Can you work these out from the model? Positions are in its coordinate system, mm. A direction names the side the tool comes from. Coordinates: 2 decimals unless noted, no trailing zeros. Loops run counter-clockwise (first coordinate to the right, second up) from the corner with the lowest first, then second, coordinate; pieces in that order, holes last.
Autodesk Inventor part; units mm, degrees
ref_plane "YZ Plane" through (0, 0, 0) normal (1, 0, 0) x (0, 1, 0)
ref_plane "XZ Plane" through (0, 0, 0) normal (0, 1, 0) x (-1, 0, 0)
ref_plane "XY Plane" through (0, 0, 0) normal (0, 0, 1) x (1, 0, 0)
sketch "Skizze1" plane through (0, 0, 0) normal (0, 0, 1) x (1, 0, 0)
  line L0 (48.8, -48.8) -> (-48.8, -48.8)
  line L1 (-48.8, -48.8) -> (-48.8, 48.8)
  line L2 (-48.8, 48.8) -> (48.8, 48.8)
  line L3 (48.8, 48.8) -> (48.8, -48.8)
  line L4 (48.8, -48.8) -> (-48.8, 48.8) construction
  line L5 (-48.8, -48.8) -> (48.8, 48.8) construction
  line L6 (-50, 50) -> (50, 50) construction
  line L7 (50, 50) -> (50, -50) construction
  line L8 (50, -50) -> (-50, -50) construction
  line L9 (-50, -50) -> (-50, 50) construction
  line L10 (-50, 50) -> (50, -50) construction
  line L11 (50, 50) -> (-50, -50) construction
  line L12 (47.75, -47.75) -> (-47.75, -47.75)
  line L13 (-47.75, -47.75) -> (-47.75, 47.75)
  line L14 (-47.75, 47.75) -> (47.75, 47.75)
  line L15 (47.75, 47.75) -> (47.75, -47.75)
  line L16 (47.75, -47.75) -> (-47.75, 47.75) construction
  line L17 (-47.75, -47.75) -> (47.75, 47.75) construction
  circle A0 centre (0, 0) radius 15 construction
  line L18 (-50, 50) -> (-39.5, 50) construction
  line L19 (-39.5, 50) -> (-39.5, 31.5) construction
  line L20 (-39.5, 31.5) -> (-50, 31.5) construction
  line L21 (-50, 31.5) -> (-50, 50) construction
  line L22 (50, 50) -> (39.5, 50) construction
  line L23 (39.5, 50) -> (39.5, 31.5) construction
  line L24 (39.5, 31.5) -> (50, 31.5) construction
  line L25 (50, 31.5) -> (50, 50) construction
  line L26 (-50, -50) -> (-39.5, -50) construction
  line L27 (-39.5, -50) -> (-39.5, -31.5) construction
  line L28 (-39.5, -31.5) -> (-50, -31.5) construction
  line L29 (-50, -31.5) -> (-50, -50) construction
  line L30 (50, -50) -> (39.5, -50) construction
  line L31 (39.5, -50) -> (39.5, -31.5) construction
  line L32 (39.5, -31.5) -> (50, -31.5) construction
  line L33 (50, -31.5) -> (50, -50) construction
  line L34 (-39.5, 47.75) -> (39.5, 47.75)
  line L35 (39.5, 47.75) -> (39.5, 45.75)
  line L36 (39.5, 45.75) -> (-39.5, 45.75)
  line L37 (-39.5, 45.75) -> (-39.5, 47.75)
  line L38 (47.75, 31.5) -> (45.75, 31.5)
  line L39 (45.75, 31.5) -> (45.75, -31.5)
  line L40 (45.75, -31.5) -> (47.75, -31.5)
  line L41 (47.75, -31.5) -> (47.75, 31.5)
  line L42 (39.5, -47.75) -> (-39.5, -47.75)
  line L43 (-39.5, -47.75) -> (-39.5, -45.75)
  line L44 (-39.5, -45.75) -> (39.5, -45.75)
  line L45 (39.5, -45.75) -> (39.5, -47.75)
  line L46 (-47.75, -31.5) -> (-45.75, -31.5)
  line L47 (-45.75, -31.5) -> (-45.75, 31.5)
  line L48 (-45.75, 31.5) -> (-47.75, 31.5)
  line L49 (-47.75, 31.5) -> (-47.75, -31.5)
  line L50 (-39.5, 45.75) -> (-39.5, 31.5)
  line L51 (-45.75, 31.5) -> (-39.5, 31.5)
  line L52 (39.5, 45.75) -> (39.5, 31.5)
  line L53 (39.5, 31.5) -> (45.75, 31.5)
  line L54 (45.75, -31.5) -> (39.5, -31.5)
  line L55 (39.5, -31.5) -> (39.5, -45.75)
  line L56 (-39.5, -45.75) -> (-39.5, -31.5)
  line L57 (-45.75, -31.5) -> (-39.5, -31.5)
  line L58 (-45.75, -29.5) -> (-37.5, -29.5)
  line L59 (-37.5, -29.5) -> (-37.5, -45.75)
  line L60 (45.75, -29.5) -> (37.5, -29.5)
  line L61 (37.5, -29.5) -> (37.5, -45.75)
  line L62 (37.5, 45.75) -> (37.5, 29.5)
  line L63 (37.5, 29.5) -> (45.75, 29.5)
  line L64 (-37.5, 45.75) -> (-37.5, 29.5)
  line L65 (-37.5, 29.5) -> (-45.75, 29.5)
  line L66 (-39.5, 45.75) -> (-37.5, 45.75)
  line L67 (-45.75, 29.5) -> (-45.75, 31.5)
  line L68 (37.5, 45.75) -> (39.5, 45.75)
  line L69 (45.75, 29.5) -> (45.75, 31.5)
  line L70 (45.75, -29.5) -> (45.75, -31.5)
  line L71 (37.5, -45.75) -> (39.5, -45.75)
  line L72 (-39.5, -45.75) -> (-37.5, -45.75)
  line L73 (-45.75, -31.5) -> (-45.75, -29.5)
  point P0 (0, 0)
  point P1 (0, 0)
  point P2 (-10.6066, 10.6066)
  point P3 (10.6066, 10.6066)
  point P4 (10.6066, -10.6066)
  point P5 (-10.6066, -10.6066)
  point P6 (-44, 44)
  point P7 (44, 44)
  point P8 (44, -44)
  point P9 (-44, -44)
  dimension "d0" = 97.6
  dimension "d55" = 30
  dimension "d61" = 100
  dimension "d62" = 95.5
  dimension "d63" = 18.5
  dimension "d64" = 10.5
  dimension "d65" = 2
  dimension "d67" = 6
extrude "Extrusion1" add sketch "Skizze1" against normal blind 2 contours L0 L1 L2 L3 | L12 L45 L55 L54 L40 L15 | L12 L43 L44 L45 | L40 L39 L38 L15 | L12 L13 L46 L57 L56 L43 | L44 L61 L60 L39 L54 L55 | L38 L53 L52 L35 L14 L15 | L56 L57 L47 L58 L59 L44 | L44 L59 L58 L47 L65 L64 L36 L62 L63 L39 L60 L61 | L39 L63 L62 L36 L52 L53 | L13 L48 L47 L46 | L35 L36 L37 L14 | L13 L14 L37 L50 L51 L48 | L51 L50 L36 L64 L65 L47
hole "Bohrung1" at (-10.6066, 10.6066, 0) at (10.6066, 10.6066, 0) at (-10.6066, -10.6066, 0) at (10.6066, -10.6066, 0) at (-44, 44, 0) at (44, 44, 0) at (44, -44, 0) at (-44, -44, 0) direction (0, 0, -1) diameter 3.4 end through all
extrude "Extrusion4" add sketch "Skizze1" along normal blind 2 contours L12 L43 L44 L45 | L40 L39 L38 L15 | L44 L61 L60 L39 L54 L55 | L56 L57 L47 L58 L59 L44 | L39 L63 L62 L36 L52 L53 | L13 L48 L47 L46 | L35 L36 L37 L14 | L51 L50 L36 L64 L65 L47
sketch "Skizze2" plane through (0, 0, -2) normal (0, 0, -1) x (-1, 0, 0)
  line L0 (-50, -50) -> (50, -50) construction
  line L1 (50, -50) -> (50, 50) construction
  line L2 (50, 50) -> (-50, 50) construction
  line L3 (-50, 50) -> (-50, -50) construction
  line L4 (-50, -50) -> (50, 50) construction
  line L5 (50, -50) -> (-50, 50) construction
  circle A0 centre (0, 0) radius 20 construction
  line L6 (0, 20) -> (0, 23)
  arc A1 (14.1421, 14.1421) -> (0, 20) centre (0, 0) ccw
  arc A2 (16.2635, 16.2635) -> (0, 23) centre (0, 0) ccw
  line L7 (14.1421, 14.1421) -> (16.2635, 16.2635)
  line L8 (-5, -25) -> (5, -25)
  line L9 (5, -25) -> (5, -30)
  line L10 (5, -30) -> (-5, -30)
  line L11 (-5, -30) -> (-5, -25)
  line L12 (-5, -25) -> (5, -30) construction
  line L13 (5, -25) -> (-5, -30) construction
  point P0 (0, 0)
  point P1 (0, 0)
  point P2 (0, -27.5)
  point P3 (0, -27.5)
  dimension "d45" = 100
  dimension "d46" = 100
  dimension "d47" = 40
  dimension "d53" = 3
  dimension "d54" = 45
  dimension "d57" = 10
  dimension "d58" = 5
  dimension "d59" = 25
extrude "Extrusion5" cut sketch "Skizze2" against normal through all
properties part number "DayLightGlow_BaseCover"
(1) If we mould it in two halves opening along Y, with no side actions, what happens to faces 3 (the flat face through (-40, 33, 0)), 4 (the cylindrical face through (-42.97, -42.65, -1.01))? For each: released by +Y, released by -Y, zero draft, split by the parting line, or undercut.
Check values:
face 3: zero draft
face 4: undercut
(2) I'm going to push flat-ended pins straight in: pin 1 (1 mm diameter, centred on x = -1.5, z = 1, fed in from -Y); pin 2 (1 mm diameter, centred on y = -13.5, z = 1.5, fed in from -X); pin 3 (0.6 mm diameter, centred on y = -34, z = 1, fed in from +X). Where does each tip first touch, or does it pass through?
Check values:
pin 1: stops at y = -47.75
pin 2: stops at x = -47.75
pin 3: stops at x = 39.5
(3) Which directions (+Z, -Z, +X, -X, +Y, -Y) give clear straight access to the entire face, cutting with the end or side of a thin tool? Please do faces 1 (the cylindrical face through (-7.755, 18.435, -1.014)), 2 (the flat face through (0, 46, 2)).
Check values:
face 1: +Z, -Z
face 2: +Z, +X, -X, +Y, -Y
(4) If I drill on probe 1 along Y at (x, z) = (-44, -0.5); probe 2 along Y at (x, z) = (-11, -0.85), over which ranges is the centre line in solid material (lowest first)?
Check values:
probe 1: y = -48.8 to -45.7, -42.3 to 42.3, 45.7 to 48.8
probe 2: y = -48.8 to -12.26, -8.95 to 8.95, 12.26 to 16.7, 20.2 to 48.8
(5) I want a section at C-C on y = -44. Write out the boundary of the cut face in (x, z), then the cut area to 3 significant figures.
Check values:
outline: (-48.8, -2) - (-45.7, -2) - (-45.7, 0) - (-48.8, 0) - close; (-42.3, -2) - (42.3, -2) - (42.3, 0) - (39.5, 0) - (39.5, 2) - (37.5, 2) - (37.5, 0) - (-37.5, 0) - (-37.5, 2) - (-39.5, 2) - (-39.5, 0) - (-42.3, 0) - close; (45.7, -2) - (48.8, -2) - (48.8, 0) - (45.7, 0) - close
area: 190 mm2
(6) I want a section at A-A on x = -44. Write out the boundary of the cut face in (y, z), then the cut area to 3 significant figures.
Check values:
outline: (-48.8, -2) - (-45.7, -2) - (-45.7, 0) - (-48.8, 0) - close; (-42.3, -2) - (42.3, -2) - (42.3, 0) - (31.5, 0) - (31.5, 2) - (29.5, 2) - (29.5, 0) - (-29.5, 0) - (-29.5, 2) - (-31.5, 2) - (-31.5, 0) - (-42.3, 0) - close; (45.7, -2) - (48.8, -2) - (48.8, 0) - (45.7, 0) - close
area: 190 mm2
(7) I want a section at B-B on z = 1.1. Write out the boundary of the cut face in (x, y), then the cut area to 3 significant figures.
Check values:
outline: (-47.75, -31.5) - (-39.5, -31.5) - (-39.5, -47.75) - (39.5, -47.75) - (39.5, -31.5) - (47.75, -31.5) - (47.75, 31.5) - (39.5, 31.5) - (39.5, 47.75) - (-39.5, 47.75) - (-39.5, 31.5) - (-47.75, 31.5) - close; hole (-45.75, -29.5) - (-37.5, -29.5) - (-37.5, -45.75) - (37.5, -45.75) - (37.5, -29.5) - (45.75, -29.5) - (45.75, 29.5) - (37.5, 29.5) - (37.5, 45.75) - (-37.5, 45.75) - (-37.5, 29.5) - (-45.75, 29.5) - close
area: 748 mm2
(8) I want a section at D-D on x = -26. Write out the boundary of the cut face in (y, z), then the cut area to 3 significant figures.
Check values:
outline: (-48.8, -2) - (48.8, -2) - (48.8, 0) - (47.75, 0) - (47.75, 2) - (45.75, 2) - (45.75, 0) - (-45.75, 0) - (-45.75, 2) - (-47.75, 2) - (-47.75, 0) - (-48.8, 0) - close
area: 203 mm2
